Input: dimensioned drawing with shaded views. Units: mm. Origin: part minimum x, y, z. A direction names the side the tool comes from. Round coordinates to 2 decimals unless told otherwise and drop trailing zeros. Order: outer loops, then holes, each group sorted by start corner. A loop starts at its lowest first (then second) coordinate and runs counter-clockwise, first axis right, second up.
Item 1: First-contact query: pin 1 (2.5 mm diameter, centred on y = 2, z = 21, fed in from -X). Flat tip, straight axial feed; report the tip coordinate or a pass-through.
Item 2: Reachability of the marked faces 1 and 2 from +Z, -Z, +X, -X, +Y, -Y: full face, straight path, thin tool, end or side. Return the list, or none.
Item 3: Mould query, pull axis Z, two halves, no side actions, for the marked faces 3, 4, 5 and 6. Classes: released by +Z, released by -Z, zero draft, split by the parting line, or undercut.
Item 4: Line query: L1, parallel to X at y = 1.65, z = 5; L2, parallel to X at y = 3.05, z = 19.75 (1 decimal); L3, parallel to Z at x = 3.75, y = 0.4 (1 decimal). Output: solid intervals per line, ascending.
Item 5: Cut plane C-C on x = 25. Output: boundary loops of the cut face in (y, z).
Item 6: Cut plane D-D on z = 9.5. Output: boundary loops of the cut face in (x, y).
Item 7: Cut plane A-A on z = 5. Output: boundary loops of the cut face in (x, y).
Item 8: Cut plane B-B on y = 4.15. Give the number of separate pieces and of enclosed holes in the cut face, then the cut area to 3 significant figures.
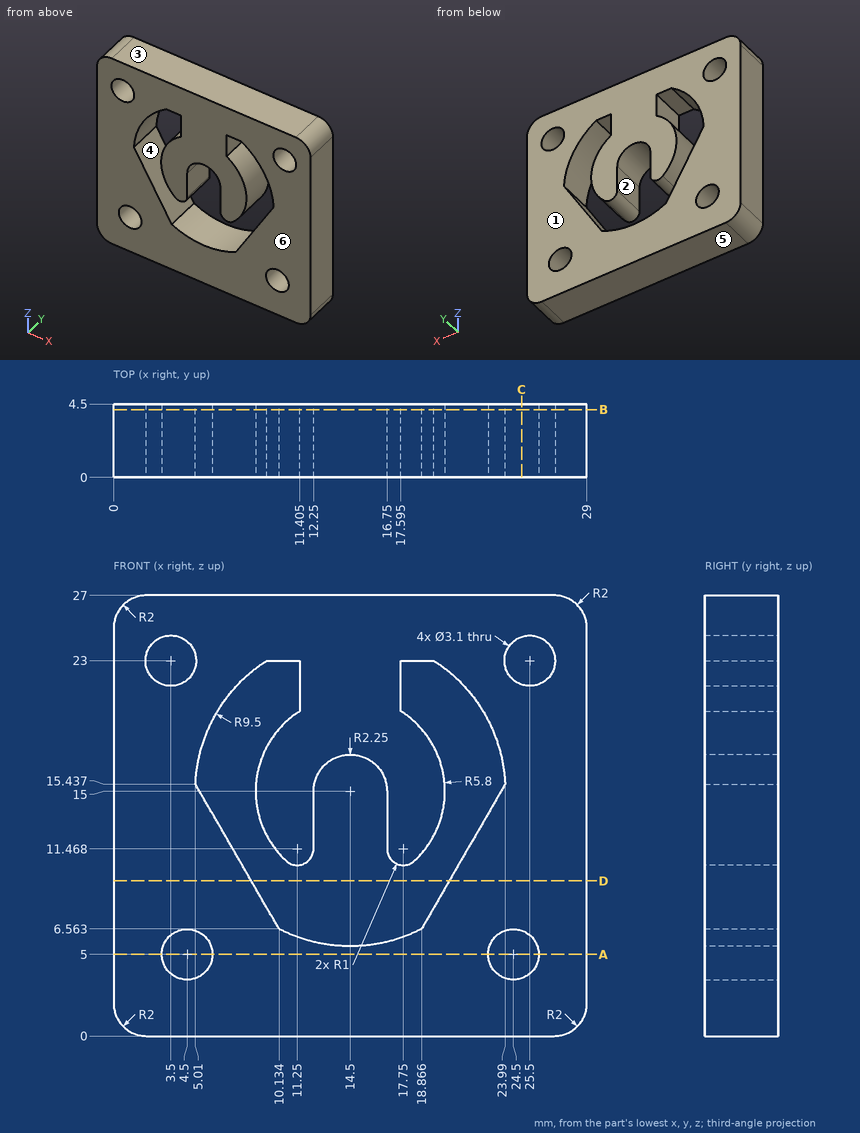
From the geometry:
1. pin 1: stops at x = 0
2. face 1: +Z, -Z, +X, -X, +Y
2. face 2: +Y, -Y
3. face 3: released by +Z
3. face 4: undercut
3. face 5: released by -Z
3. face 6: zero draft
4. L1: x = 0 to 2.95, 6.05 to 22.95, 26.05 to 29
4. L2: x = 0 to 6.3, 11.2 to 17.8, 22.7 to 29
4. L3: z = 0 to 3.6, 6.4 to 21.5, 24.5 to 27
5. outline: (0, 0) - (4.5, 0) - (4.5, 3.53) - (0, 3.53) - close; (0, 6.47) - (4.5, 6.47) - (4.5, 21.53) - (0, 21.53) - close; (0, 24.47) - (4.5, 24.47) - (4.5, 27) - (0, 27) - close
6. outline: (0, 0) - (8.44, 0) - (8.44, 4.5) - (0, 4.5) - close; (20.56, 0) - (29, 0) - (29, 4.5) - (20.56, 4.5) - close
7. outline: (0, 0) - (2.95, 0) - (2.95, 4.5) - (0, 4.5) - close; (6.05, 0) - (22.95, 0) - (22.95, 4.5) - (6.05, 4.5) - close; (26.05, 0) - (29, 0) - (29, 4.5) - (26.05, 4.5) - close
8. separate pieces: 1
8. enclosed holes: 5
8. area: 583 mm2
